from build123d import *

# Parameters (mm, degrees)
SKETCH_1_W          = 50
SKETCH_1_H          = 30
SKETCH_1_R          = 1
EXTRUDE_1_DEPTH     = 45.03
SKETCH_2_W          = 46
SKETCH_2_H          = 41.03
CUT_EXTRUDE_1_DEPTH = 45.03
SKETCH_3_R          = 1
CUT_EXTRUDE_2_DEPTH = 45.03
SKETCH_4_W          = 4
SKETCH_4_H          = 41.03
CUT_EXTRUDE_3_DEPTH = 26


with BuildPart() as part:
    # 草图1 → 凸台-拉伸1 (new body)
    with BuildSketch(Plane.XY):
        Rectangle(SKETCH_1_W, SKETCH_1_H)
        with Locations((-23, -13)):
            Circle(SKETCH_1_R, mode=Mode.SUBTRACT)
        with Locations((-23, 13)):
            Circle(SKETCH_1_R, mode=Mode.SUBTRACT)
    extrude(amount=EXTRUDE_1_DEPTH)

    # 草图2 → 切除-拉伸1 (cut)
    with BuildSketch(Plane(origin=(0, 15, 0), x_dir=(1, 0, 0), z_dir=(0, 1, 0))):
        with Locations((-2, -22.515)):
            Rectangle(SKETCH_2_W, SKETCH_2_H)
    extrude(amount=-CUT_EXTRUDE_1_DEPTH, mode=Mode.SUBTRACT)

    # 草图3 → 切除-拉伸2 (cut)
    with BuildSketch(Plane.XY.offset(45.03)):
        with Locations((23, -13)):
            Circle(SKETCH_3_R)
    extrude(amount=-CUT_EXTRUDE_2_DEPTH, mode=Mode.SUBTRACT)

    # 草图4 → 切除-拉伸3 (cut)
    with BuildSketch(Plane(origin=(0, 15, 0), x_dir=(1, 0, 0), z_dir=(0, 1, 0))):
        with Locations((23, -22.515)):
            Rectangle(SKETCH_4_W, SKETCH_4_H)
    extrude(amount=-CUT_EXTRUDE_3_DEPTH, mode=Mode.SUBTRACT)


solid = part.part
Verification items for the finished model (mm, model axes). A direction names the side the tool comes from. Coordinates: 2 decimals unless noted, no trailing zeros. Order: outer loops, then holes, each group sorted by start corner. A loop starts at its lowest first (then second) coordinate and runs counter-clockwise, first axis right, second up.
1. Go/stop test with flat-tipped pins: pin 1 Ø3 at (x, z) = (23.5, 29.5) entering from +Y; pin 2 Ø2.5 at (x, y) = (-23, -13) entering from +Z; pin 3 Ø12 at (y, z) = (-8, 25) entering from -X; pin 4 Ø1.2 at (x, y) = (-23, 13) entering from +Z. Record where each tip stops, or that it passes through.
Results found:
pin 1: stops at y = -11
pin 2: stops at z = 45.03
pin 3: stops at x = 21
pin 4: passes through
2. Scan lines: line 1 (Y direction, x = -23, z = 44.4); line 2 (Z direction, x = 10.5, y = -9.5); line 3 (X direction, y = 13, z = 44.6). Record each from-to range of solid material in increasing order.
Results found:
line 1: y = -15 to -14, -12 to 12, 14 to 15
line 2: z = 0 to 2, 43.03 to 45.03
line 3: x = -25 to -24, -22 to 25
3. Set-up check for faces 1 (the face through (23, -11, 22)), 2 (the face through (22, -15, 22)): record each of +Z, -Z, +X, -X, +Y, -Y from which the full face is reachable in a straight line by a thin tool's end or side.
Results found:
face 1: +X, -X, +Y
face 2: +Z, -Z, +X, -X, -Y
4. Sectioned sample at C-C, the plane z = 30. Record the cut outline in (x, y), and give its area (3 significant figures).
Results found:
outline: (21, -15) - (25, -15) - (25, -11) - (21, -11) - close; hole circle Ø2 at (23, -13)
area: 12.9 mm2
5. Sectioned sample at B-B, the plane x = 23. Record the cut outline in (y, z).
Results found:
outline: (-15, 0) - (-14, 0) - (-14, 45.03) - (-15, 45.03) - close; (-12, 0) - (15, 0) - (15, 2) - (-11, 2) - (-11, 43.03) - (15, 43.03) - (15, 45.03) - (-12, 45.03) - close
6. Sectioned sample at A-A, the plane y = 13. Record the cut outline in (x, z).
Results found:
outline: (-25, 0) - (-24, 0) - (-24, 2) - (-25, 2) - close; (-25, 43.03) - (-24, 43.03) - (-24, 45.03) - (-25, 45.03) - close; (-22, 0) - (25, 0) - (25, 2) - (-22, 2) - close; (-22, 43.03) - (25, 43.03) - (25, 45.03) - (-22, 45.03) - close
7. Sectioned sample at D-D, the plane x = -23. Record the cut outline in (y, z), and give its area (3 significant figures).
Results found:
outline: (-15, 0) - (-14, 0) - (-14, 2) - (-15, 2) - close; (-15, 43.03) - (-14, 43.03) - (-14, 45.03) - (-15, 45.03) - close; (-12, 0) - (12, 0) - (12, 2) - (-12, 2) - close; (-12, 43.03) - (12, 43.03) - (12, 45.03) - (-12, 45.03) - close; (14, 0) - (15, 0) - (15, 2) - (14, 2) - close; (14, 43.03) - (15, 43.03) - (15, 45.03) - (14, 45.03) - close
area: 104 mm2
8. Release check for a two-part mould opening along X. For faces 3 (the face through (-23, 12, 1)), 4 (the face through (23, -14, 23)), 5 (the face through (0, 15, 1)), 6 (the face through (21, -13, 23)) record: +X half, -X half, draft (parallel to the pull), parting line (faces both ways), or undercut.
Results found:
face 3: undercut
face 4: undercut
face 5: draft
face 6: -X half
